Could you check a few things on this model? Use its own coordinates, in mm. Coordinates: 2 decimals unless noted, no trailing zeros. Loops run counter-clockwise (first coordinate to the right, second up) from the corner with the lowest first, then second, coordinate; pieces in that order, holes last. Notation, with made-up numbers: (-35.75, 34) -> (-0.75, 34) arc R33 cw to (-0.75, 68) -> close; hole circle Ø2 at (37, 43). An arc over 180 degrees is marked (long way). One line per question, with ' | ' between items. Start each with the question number.
(1) Suppose I cut it at A-A (z = 368.5). Please give me the cut outline in (x, y).
(2) Suppose I cut it at C-C (x = 1.4). Give the number of separate pieces and of enclosed holes in the cut face, plus the area to 3 significant figures.
(3) Suppose I cut it at B-B (z = 300.5). Please give me the cut outline in (x, y).
(4) I'm going to push flat-ended pins straight in: pin 1 Ø3 at (x, y) = (1, 88) entering from -Z; pin 2 Ø2 at (x, z) = (1.5, 354.5) entering from -Y; pin 3 Ø2.5 at (x, y) = (2, 116.5) entering from -Z. Where does each tip first touch, or does it pass through?
(5) If we mould it in two halves opening along Y, with no side actions, what happens to faces 1 (the face through (5, 58, 197)), 2 (the face through (2.46, 67.85, 208.01))? For each: pulls with the +Y half, pulls with the -Y half, needs draft (parallel to the pull), parting line crosses it, or undercut.
(6) Suppose I cut it at D-D (z = 76). Please give me the cut outline in (x, y), plus the area to 3 significant figures.
(7) If I drill on line 1 along Y through (x, z) = (2.65, 224); line 2 along Z through (x, y) = (3.75, 78); line 3 along Y through (x, z) = (3.8, 334), over which ranges is the centre line in solid material (lowest first)?
```python
from build123d import *

# Parameters (mm, degrees)
SKETCH_1_R      = 5
SKETCH_1_R_2    = 4
SKETCH_1_R_3    = 2.5
EXTRUDE_1_DEPTH = 5


with BuildPart() as part:
    # 草图1 → 凸台-拉伸1 (new body)
    with BuildSketch(Plane(origin=(0, 0, 0), x_dir=(0, 0, -1), z_dir=(1, 0, 0))):
        Polygon((-400, 82.5), (-400, 115), (-345, 115), (-345, 120), (-295, 120), (-295, 115), (-105, 115), (-105, 120), (-55, 120), (-55, 115), (0, 115), (0, 82.5), (5, 82.5), (5, 32.5), (0, 32.5), (0, 0), (-55, 0), (-55, -5), (-105, -5), (-105, 0), (-295, 0), (-295, -5), (-345, -5), (-345, 0), (-400, 0), (-400, 32.5), (-405, 32.5), (-405, 82.5), align=None)
        with Locations((-368.5, 85)):
            Circle(SKETCH_1_R, mode=Mode.SUBTRACT)
        with Locations((-368.5, 21)):
            Circle(SKETCH_1_R_2, mode=Mode.SUBTRACT)
        with Locations((-31.5, 21)):
            Circle(SKETCH_1_R_2, mode=Mode.SUBTRACT)
        with Locations((-31.5, 85)):
            Circle(SKETCH_1_R, mode=Mode.SUBTRACT)
        with Locations((-200, 10)):
            Circle(SKETCH_1_R_3, mode=Mode.SUBTRACT)
        with Locations((-170, 10)):
            Circle(SKETCH_1_R_3, mode=Mode.SUBTRACT)
        with Locations((-140, 10)):
            Circle(SKETCH_1_R_3, mode=Mode.SUBTRACT)
        with Locations((-230, 10)):
            Circle(SKETCH_1_R_3, mode=Mode.SUBTRACT)
        with Locations((-260, 10)):
            Circle(SKETCH_1_R_3, mode=Mode.SUBTRACT)
        with BuildLine():
            Line((-340, 50), (-60, 50))
            ThreePointArc((-60, 50), (-52.928932188, 47.071067812), (-50, 40))
            Line((-50, 40), (-50, 30))
            ThreePointArc((-50, 30), (-52.928932188, 22.928932188), (-60, 20))
            Line((-60, 20), (-340, 20))
            ThreePointArc((-340, 20), (-347.071067812, 22.928932188), (-350, 30))
            Line((-350, 30), (-350, 40))
            ThreePointArc((-350, 40), (-347.071067812, 47.071067812), (-340, 50))
        make_face(mode=Mode.SUBTRACT)
        with BuildLine():
            Line((-340, 95), (-315, 95))
            ThreePointArc((-315, 95), (-307.928932188, 92.071067812), (-305, 85))
            Line((-305, 85), (-305, 75))
            ThreePointArc((-305, 75), (-307.928932188, 67.928932188), (-315, 65))
            Line((-315, 65), (-340, 65))
            ThreePointArc((-340, 65), (-347.071067812, 67.928932188), (-350, 75))
            Line((-350, 75), (-350, 85))
            ThreePointArc((-350, 85), (-347.071067812, 92.071067812), (-340, 95))
        make_face(mode=Mode.SUBTRACT)
        with BuildLine():
            Line((-50, 85), (-50, 75))
            ThreePointArc((-50, 75), (-52.928932188, 67.928932188), (-60, 65))
            Line((-60, 65), (-85, 65))
            ThreePointArc((-85, 65), (-92.071067812, 67.928932188), (-95, 75))
            Line((-95, 75), (-95, 85))
            ThreePointArc((-95, 85), (-92.071067812, 92.071067812), (-85, 95))
            Line((-85, 95), (-60, 95))
            ThreePointArc((-60, 95), (-52.928932188, 92.071067812), (-50, 85))
        make_face(mode=Mode.SUBTRACT)
        with BuildLine():
            Line((-185, 65), (-165, 65))
            ThreePointArc((-165, 65), (-157.928932188, 67.928932188), (-155, 75))
            Line((-155, 75), (-155, 85))
            ThreePointArc((-155, 85), (-157.928932188, 92.071067812), (-165, 95))
            Line((-165, 95), (-185, 95))
            ThreePointArc((-185, 95), (-192.071067812, 92.071067812), (-195, 85))
            Line((-195, 85), (-195, 75))
            ThreePointArc((-195, 75), (-192.071067812, 67.928932188), (-185, 65))
        make_face(mode=Mode.SUBTRACT)
        with BuildLine():
            Line((-235, 65), (-215, 65))
            ThreePointArc((-215, 65), (-207.928932188, 67.928932188), (-205, 75))
            Line((-205, 75), (-205, 85))
            ThreePointArc((-205, 85), (-207.928932188, 92.071067812), (-215, 95))
            Line((-215, 95), (-235, 95))
            ThreePointArc((-235, 95), (-242.071067812, 92.071067812), (-245, 85))
            Line((-245, 85), (-245, 75))
            ThreePointArc((-245, 75), (-242.071067812, 67.928932188), (-235, 65))
        make_face(mode=Mode.SUBTRACT)
    extrude(amount=EXTRUDE_1_DEPTH)


solid = part.part
```
Checks:
1) outline: (0, 0) -> (5, 0) -> (5, 17) -> (0, 17) -> close; (0, 25) -> (5, 25) -> (5, 80) -> (0, 80) -> close; (0, 90) -> (5, 90) -> (5, 115) -> (0, 115) -> close
2) separate pieces: 1 | enclosed holes: 14 | area: 33,500 mm^2
3) outline: (0, -5) -> (5, -5) -> (5, 20) -> (0, 20) -> close; (0, 50) -> (5, 50) -> (5, 120) -> (0, 120) -> close
4) pin 1: stops at z = 0 | pin 2: stops at y = 0 | pin 3: stops at z = 55
5) face 1: needs draft | face 2: undercut
6) outline: (0, -5) -> (5, -5) -> (5, 20) -> (0, 20) -> close; (0, 50) -> (5, 50) -> (5, 65) -> (0, 65) -> close; (0, 95) -> (5, 95) -> (5, 120) -> (0, 120) -> close | area: 325 mm^2
7) line 1: y = 0 to 20, 50 to 65, 95 to 115 | line 2: z = -5 to 50, 95 to 155, 195 to 205, 245 to 305, 350 to 405 | line 3: y = -5 to 20, 50 to 65, 95 to 120
